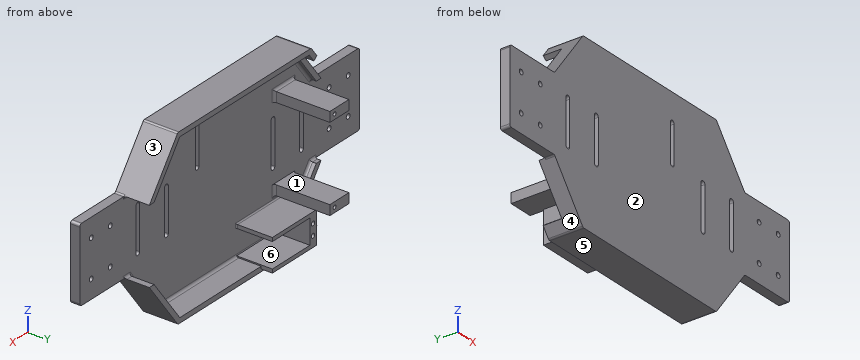
from build123d import *

# Parameters (mm, degrees)
SKETCH1_W            = 47
SKETCH1_H            = 60
SKETCH1_W_2          = 140
SKETCH1_H_2          = 140
BOSS_EXTRUDE1_DEPTH  = 7.5
SKETCH2_R            = 2
CUT_EXTRUDE1_DEPTH   = 10
BOSS_EXTRUDE2_DEPTH  = 20
CUT_EXTRUDE3_DEPTH   = 10
FILLET5_R            = 2
FILLET6_R            = 2
FILLET7_R            = 2
SKETCH12_W           = 15.204619521
SKETCH12_H           = 41.964749879
BOSS_EXTRUDE3_DEPTH  = 7.5
SKETCH13_W           = 40
SKETCH13_H           = 15
CUT_EXTRUDE4_DEPTH   = 10
SKETCH15_W           = 20
SKETCH15_H           = 8
BOSS_EXTRUDE4_DEPTH  = 45
SKETCH16_R           = 1.5
CUT_EXTRUDE5_DEPTH   = 8
FILLET9_R            = 2
FILLET9_OF_MIRROR5_R = 2
BOSS_EXTRUDE5_DEPTH  = 29
FILLET10_R           = 1
SKETCH18_R           = 1.75
CUT_EXTRUDE6_DEPTH   = 15
SKETCH19_W           = 12.583718204
SKETCH19_H           = 7.390312174
CUT_EXTRUDE7_DEPTH   = 10
FILLET11_R           = 2


with BuildPart() as part:
    # Sketch1 → Boss-Extrude1 (new body)
    with BuildSketch(Plane(origin=(0, 0, 0), x_dir=(1, 0, 0), z_dir=(0, 1, 0))):
        with Locations((-123.5, 0)):
            Rectangle(SKETCH1_W, SKETCH1_H)
        Polygon((-100, 30), (-100, -30), (-70, -70), (-70, 70), align=None)
        Rectangle(SKETCH1_W_2, SKETCH1_H_2)
        Polygon((100, 30), (100, -30), (70, -70), (70, 70), align=None)
        with Locations((123.5, 0)):
            Rectangle(SKETCH1_W, SKETCH1_H)
    extrude(amount=BOSS_EXTRUDE1_DEPTH)

    # Sketch2 → Cut-Extrude1 (cut)
    with BuildSketch(Plane(origin=(0, 7.5, 0), x_dir=(1, 0, 0), z_dir=(0, 1, 0))):
        with Locations(Location((-135, 15, 0), (0, 0, 270))):
            Circle(SKETCH2_R)
        with Locations(Location((-115, 15, 0), (0, 0, 270))):
            Circle(SKETCH2_R)
        with Locations(Location((-135, -15, 0), (0, 0, 270))):
            Circle(SKETCH2_R)
        with Locations(Location((-115, -15, 0), (0, 0, 270))):
            Circle(SKETCH2_R)
    cut_extrude1 = extrude(amount=-CUT_EXTRUDE1_DEPTH, mode=Mode.SUBTRACT)

    # Sketch8 → Boss-Extrude2 (add)
    with BuildSketch(Plane(origin=(0, 7.5, 0), x_dir=(1, 0, 0), z_dir=(0, 1, 0))):
        Polygon((-100, 30), (-70, 70), (70, 70), (100, 30), (95, 30), (68, 66), (-68, 66), (-95, 30), align=None)
        Polygon((-100, -30), (-70, -70), (70, -70), (100, -30), (95, -30), (68, -66), (-68, -66), (-95, -30), align=None)
    extrude(amount=BOSS_EXTRUDE2_DEPTH)

    # Mirror1: Cut-Extrude1 across plane
    add(cut_extrude1.mirror(Plane(origin=(0, 0, 0), x_dir=(0, 0, 1), z_dir=(1, 0, 0))), mode=Mode.SUBTRACT)

    # Sketch11 → Cut-Extrude3 (cut)
    with BuildSketch(Plane(origin=(0, 7.5, 0), x_dir=(1, 0, 0), z_dir=(0, 1, 0))):
        with BuildLine():
            Line((58, -17.5), (58, 17.5))
            ThreePointArc((58, 17.5), (56, 19.5), (54, 17.5))
            Line((54, 17.5), (54, -17.5))
            ThreePointArc((54, -17.5), (56, -19.5), (58, -17.5))
        make_face()
        with BuildLine():
            Line((84, -17.5), (84, 17.5))
            ThreePointArc((84, 17.5), (86, 19.5), (88, 17.5))
            Line((88, 17.5), (88, -17.5))
            ThreePointArc((88, -17.5), (86, -19.5), (84, -17.5))
        make_face()
        with BuildLine():
            Line((21.85, -17.5), (21.85, -47.5))
            ThreePointArc((21.85, -47.5), (23.75, -49.4), (25.65, -47.5))
            Line((25.65, -47.5), (25.65, -17.5))
            ThreePointArc((25.65, -17.5), (23.75, -15.6), (21.85, -17.5))
        make_face()
    cut_extrude3 = extrude(amount=-CUT_EXTRUDE3_DEPTH, mode=Mode.SUBTRACT)

    # Fillet5
    fillet5_edges = [part.edges().sort_by_distance(p)[0] for p in [
        (-147, 3.75, 30),
        (-147, 3.75, -30),
        (-100, 3.75, -30),
        (-70, 13.75, -70),
        (70, 13.75, -70),
        (100, 3.75, -30),
        (147, 3.75, -30),
        (147, 3.75, 30),
        (100, 3.75, 30),
        (70, 13.75, 70),
        (-70, 13.75, 70),
        (-100, 3.75, 30),
    ]]
    fillet(fillet5_edges, radius=FILLET5_R)

    # Fillet6
    fillet6_edges = [part.edges().sort_by_distance(p)[0] for p in [
        (-81.5, 7.5, -48),
        (0, 7.5, -66),
        (81.5, 7.5, -48),
        (81.5, 7.5, 48),
        (0, 7.5, 66),
        (-81.5, 7.5, 48),
    ]]
    fillet(fillet6_edges, radius=FILLET6_R)

    # Fillet7
    fillet7_edges = [part.edges().sort_by_distance(p)[0] for p in [
        (96.25, 7.5, 30),
        (-96.25, 7.5, 30),
        (-96.25, 7.5, -30),
        (96.25, 7.5, -30),
    ]]
    fillet(fillet7_edges, radius=FILLET7_R)

    # Mirror2: Cut-Extrude3 across plane
    add(cut_extrude3.mirror(Plane(origin=(0, 0, 0), x_dir=(0, 0, 1), z_dir=(1, 0, 0))), mode=Mode.SUBTRACT)

    # Sketch12 → Boss-Extrude3 (add)
    with BuildSketch(Plane(origin=(0, 7.5, 0), x_dir=(1, 0, 0), z_dir=(0, 1, 0))):
        with Locations((-23.111021673, -33.450162947)):
            Rectangle(SKETCH12_W, SKETCH12_H)
    extrude(amount=-BOSS_EXTRUDE3_DEPTH)

    # Sketch13 → Cut-Extrude4 (cut)
    with BuildSketch(Plane(origin=(-78.4, 0, 58.8), x_dir=(0.6, 0, 0.8), z_dir=(-0.8, 0, 0.6))):
        with Locations((-16, 20)):
            Rectangle(SKETCH13_W, SKETCH13_H)
    cut_extrude4 = extrude(amount=-CUT_EXTRUDE4_DEPTH, mode=Mode.SUBTRACT)

    # Mirror3: Cut-Extrude4 across plane
    add(cut_extrude4.mirror(Plane.XY), mode=Mode.SUBTRACT)

    # Sketch15 → Boss-Extrude4 (add)
    with BuildSketch(Plane(origin=(0, 7.5, 0), x_dir=(1, 0, 0), z_dir=(0, 1, 0))):
        with Locations((-67, -34)):
            Rectangle(SKETCH15_W, SKETCH15_H)
    boss_extrude4 = extrude(amount=BOSS_EXTRUDE4_DEPTH)

    # Sketch16 → Cut-Extrude5 (cut)
    with BuildSketch(Plane(origin=(0, 52.5, 0), x_dir=(1, 0, 0), z_dir=(0, 1, 0))):
        with Locations(Location((-62, -34, 0), (0, 0, 270))):
            Circle(SKETCH16_R)
    cut_extrude5 = extrude(amount=-CUT_EXTRUDE5_DEPTH, mode=Mode.SUBTRACT)

    # Fillet9
    fillet9_edges = [part.edges().sort_by_distance(p)[0] for p in [
        (-77, 7.5, 34),
    ]]
    fillet(fillet9_edges, radius=FILLET9_R)

    # Mirror5: Boss-Extrude4, Cut-Extrude5 across plane
    add(boss_extrude4.mirror(Plane.XY))
    add(cut_extrude5.mirror(Plane.XY), mode=Mode.SUBTRACT)

    # Fillet9 of Mirror5
    fillet9_of_mirror5_edges = [part.edges().sort_by_distance(p)[0] for p in [
        (-77, 7.5, -34),
    ]]
    fillet(fillet9_of_mirror5_edges, radius=FILLET9_OF_MIRROR5_R)

    # Sketch17 → Boss-Extrude5 (add)
    with BuildSketch(Plane(origin=(0, 7.5, 0), x_dir=(1, 0, 0), z_dir=(0, 1, 0))):
        Polygon((-64, 68), (-64, 42), (-17.5, 42), (-17.5, 45), (-57, 45), (-57, 65), (-17.5, 65), (-17.5, 68), align=None)
    extrude(amount=BOSS_EXTRUDE5_DEPTH)

    # Fillet10
    fillet10_edges = [part.edges().sort_by_distance(p)[0] for p in [
        (-64, 8.085786438, -65.414213562),
        (-64, 18.5, -66),
        (-64, 7.5, -53),
        (-40.75, 7.5, -42),
        (-17.5, 7.5, -43.5),
    ]]
    fillet(fillet10_edges, radius=FILLET10_R)

    # Sketch18 → Cut-Extrude6 (cut)
    with BuildSketch(Plane(origin=(0, 36.5, 0), x_dir=(1, 0, 0), z_dir=(0, 1, 0))):
        with Locations(Location((-60.25, 50.5, 0), (0, 0, 270))):
            Circle(SKETCH18_R)
        with Locations(Location((-60.25, 59.5, 0), (0, 0, 270))):
            Circle(SKETCH18_R)
    extrude(amount=-CUT_EXTRUDE6_DEPTH, mode=Mode.SUBTRACT)

    # Sketch19 → Cut-Extrude7 (cut)
    with BuildSketch(Plane.ZY.offset(64)):
        with Locations((-53.897066291, 12.195156087)):
            Rectangle(SKETCH19_W, SKETCH19_H)
    extrude(amount=-CUT_EXTRUDE7_DEPTH, mode=Mode.SUBTRACT)

    # Fillet11
    fillet11_edges = [part.edges().sort_by_distance(p)[0] for p in [
        (-68, 7.5, -38),
        (-57, 7.5, -34),
        (-57, 7.5, 34),
        (-68, 7.5, 38),
    ]]
    fillet(fillet11_edges, radius=FILLET11_R)


solid = part.part
For this review, take the finished solid that the model builds, in its own axes (mm). Face numbers are marked on the shaded views. A direction names the side the tool comes from. Give positions to 0.01 mm unless a question says otherwise; leave off trailing zeros. Loops run counter-clockwise (first coordinate to the right, second up) from the corner with the lowest first, then second, coordinate; pieces in that order, holes last. Notation, with made-up numbers: M 13.25,52.5 L 37.25,52.5 A16 ccw 37.25,59.5 Z; hole C 44,-35 d11. An arc over 180 degrees is marked long. Answer as a JSON object with one key per item and string values. Group by question number.
Q1. Add section A-A on z = -1.5. Give the boundary of the cut face in (x, y), and give its area (4 significant figures).
Q2. Insertion check: P1, Ø12, axis at x = 106, y = 7.5, coming from the -Z side; P2, Ø12, axis at x = -95.5, z = -38.5, coming from the +Y side; P3, Ø4.5, axis at x = 135, z = -15, coming from the +Y side; P4, Ø8, axis at y = 45, z = 24.5, coming from the +X side. Each pin has a flat end and moves straight along its axis. Give the tip position at first contact, or say it passes through.
Q3. Add section C-C on z = -22.5. Give the boundary of the cut face in (x, y).
Q4. Add section B-B on x = -41. Give the boundary of the cut face in (y, z).
Q5. For probe 1 along Z at (x, y) = (-60, 26); probe 2 along Z at (x, y) = (-135, 1.5); probe 3 along X at (y, z) = (3, 5), list the stretches that pass through material, from the lowest coordinate up. Write a range as [from, to].
Q6. Mouldability with a two-part tool opening along Z and no side actions: class the marked faces 1, 2, 3 and 4 as +Z half, -Z half, draft (parallel to the pull), parting line (faces both ways), or undercut.
Q7. Tool access review of the marked faces 5 and 6: name each direction out of +Z, -Z, +X, -X, +Y, -Y from which nothing blocks a thin tool from reaching the whole face with its end or side.
Checked values:
{
 "1": {"outline": "M -147,0 L -88,0 L -88,7.5 L -147,7.5 Z; M -84,0 L -58,0 L -58,7.5 L -84,7.5 Z; M -54,0 L 54,0 L 54,7.5 L -54,7.5 Z; M 58,0 L 84,0 L 84,7.5 L 58,7.5 Z; M 88,0 L 147,0 L 147,7.5 L 88,7.5 Z", "area": "2,085 mm²"},
 "2": {"P1": "z = -30.27", "P2": "y = 12.5", "P3": "y = 7.5", "P4": "through"},
 "3": {"outline": "M -147,0 L 147,0 L 147,7.5 L -147,7.5 Z"},
 "4": {"outline": "M 0,-70 L 27.5,-70 L 27.5,-68 L 36.5,-68 L 36.5,-65 L 7.77,-65 A2 cw 7.5,-64 L 7.5,-45 L 36.5,-45 L 36.5,-42 L 8.5,-42 A1 cw 7.5,-41 L 7.5,64 A2 cw 9.5,66 L 27.5,66 L 27.5,70 L 0,70 Z"},
 "5": {"probe 1": "[-70, -61.23], [-57.77, -52.23], [-48.77, -42], [-38, -30], [30, 38], [66, 70]", "probe 2": "[-30, -17], [-13, 13], [17, 30]", "probe 3": "[-147, -88], [-84, -58], [-54, 54], [58, 84], [88, 147]"},
 "6": {"face 1": "undercut", "face 2": "draft", "face 3": "+Z half", "face 4": "-Z half"},
 "7": {"face 5": "-Z, +X, -X, +Y, -Y", "face 6": "+Y"}
}
